Autodesk Inventor part; units mm, degrees
ref_plane "Start Plane" through (0, 0, -4.19) normal (0, 0, 1) x (1, 0, 0)
ref_plane "End Plane" through (0, 0, 265.8983) normal (0, 0, 1) x (1, 0, 0)
ref_plane "Work Plane4" through (10.0091, 3.6912, 287.2885) normal (-0.8617, -0.3178, 0.3957) x (0.468, -0.1962, 0.8617)
ref_plane "Start Plane" through (0, 0, -4.19) normal (0, 0, 1) x (1, 0, 0)
ref_plane "End Plane" through (0, 0, 265.8983) normal (0, 0, 1) x (1, 0, 0)
sketch "Sketch" plane through (0, 0, 0) normal (0, 0, 1) x (1, 0, 0)
  circle A0 centre (0, 0) radius 6.9342
  circle A1 centre (0, 0) radius 10.668
  dimension "d0" = 21.336
  dimension "d1" = 3.7338
extrude "Body" add sketch "Sketch" along normal up to surface (270.0883 mm away) from surface at -4.19
sketch "Sketch3" plane through (0, 0, 0) normal (0, 0, 1) x (1, 0, 0)
  line L0 (0, 0) -> (10, 0)
ref_plane "Work Plane3" through (0, 0, 0) normal (0, -1, 0) x (1, 0, 0)
sketch "Sketch4" plane through (0, 0, 0) normal (0, -1, 0) x (1, 0, 0)
  line L0 (-2, -4.19) -> (12, -4.19)
  line L1 (-2, 265.8983) -> (12, 265.8983)
  dimension "d7" = 270.0883
ref_plane "Work Plane4" through (10.0091, 3.6912, 287.2885) normal (-0.8617, -0.3178, 0.3957) x (0.468, -0.1962, 0.8617)
split "Split1" plane through (10.0091, 3.6912, 287.2885) removes the side toward (-0.8617, -0.3178, 0.3957)
ref_plane "Work Plane5" through (-7.3135, -7.7665, 273.0637) normal (0.4817, 0.5116, 0.7115) x (0.8644, -0.144, -0.4817)
split "Split2" plane through (-7.3135, -7.7665, 273.0637) removes the side toward (0.4817, 0.5116, 0.7115)
ref_plane "Work Plane6" through (7.4386, -7.6468, 269.3352) normal (-0.3751, 0.3856, 0.843) x (0.9237, 0.0785, 0.3751)
split "Split3" plane through (7.4386, -7.6468, 269.3352) removes the side toward (-0.3751, 0.3856, 0.843)
ref_plane "Work Plane7" through (-7.3135, -7.7665, -30.4674) normal (0.647, 0.6871, -0.3305) x (0.3747, -0.664, -0.647)
split "Split4" plane through (-7.3135, -7.7665, -30.4674) removes the side toward (0.647, 0.6871, -0.3305)
ref_plane "Work Plane8" through (-0.1362, -10.6671, -7.916) normal (0.0076, 0.5958, -0.8031) x (0.9997, -0.023, -0.0076)
split "Split5" plane through (-0.1362, -10.6671, -7.916) removes the side toward (0.0076, 0.5958, -0.8031)
ref_plane "Work Plane9" through (10.325, 2.6834, -10.2024) normal (-0.6689, -0.1739, -0.7227) x (-0.6137, -0.4194, 0.6689)
split "Split6" plane through (10.325, 2.6834, -10.2024) removes the side toward (-0.6689, -0.1739, -0.7227)
equation "\"d0\" = G_H"
equation "\"d1\" = G_T"
equation "\"d2\" = G_L"
equation "\"G_H\" = 21.336"
equation "\"G_T\" = 3.7338"
equation "\"G_L\" = 270.08826"
equation "\"G_OFFSET_START\" = 4.18997"
equation "\"G_OFFSET_END\" = 3.36995"
equation "\"d4\" = -G_OFFSET_START"
equation "\"d5\" = G_OFFSET_END + B_L"
equation "\"B_L\" = 262.52833"
properties part number "ANSI - 1/2 x 0.147 - 10.633" material "Steel, Mild"
Work out the finished part from the listing and answer in its coordinate system (mm). Round coordinates to 2 decimals unless told otherwise and drop trailing zeros. Write each loop counter-clockwise with the first axis right and the second up, starting at its lowest first coordinate (ties: lowest second). Pieces come first, ordered by that corner, then holes. Notation, with made-up numbers: (24.25, 40.25) - (49.25, 40.25) arc R6 ccw to (49.25, 45.25) - close; hole circle Ø1 at (70.25, 45.5). An arc over 180 degrees is marked (long way). Return JSON: item names as keys, results as strings. Group by question number.
Q1. Each of these flat-tipped pins is pushed along its axis until it touches: pin 1 Ø3 at (x, z) = (5, 110) entering from -Y; pin 2 Ø10 at (x, y) = (8.5, -2) entering from +Z; pin 3 Ø4 at (y, z) = (-6, 106.5) entering from +X. Where does it stop, or does it pass through?
Q2. The part is cut by section B-B on z = 49. Write down the section's boundary in (x, y).
Q3. The part is cut by section A-A on y = 0. Write down the section's boundary in (x, z), then the cut area to 3 significant figures.
Q4. The mould has two halves that part along Y. Classify faces 1 (the cylindrical face through (3.728, -5.847, 129.125)), 2 (the flat face through (-5.766, -4.613, 246.266)), 3 (the cylindrical face through (10.175, -3.204, 128.963)): released by +Y, released by -Y, zero draft, split by the parting line, or undercut.
Q5. Find the intervals of material crossed by L1, parallel to X at y = 0, z = 65; L2, parallel to Z at x = 4.5, y = -7.25, in increasing order.
Solved:
{
 "1": {"pin 1": "y = -10.08", "pin 2": "z = 263.15", "pin 3": "x = 9.89"},
 "2": {"outline": "circle Ø21.34 at (0, 0); hole circle Ø13.87 at (0, 0)"},
 "3": {"outline": "(-10.67, 9.87) - (-6.93, 6.42) - (-6.93, 247.43) - (-10.67, 239.3) - close; (6.93, 13.57) - (10.67, 20.88) - (10.67, 255.31) - (6.93, 257.83) - close", "area": "1,770 mm²"},
 "4": {"face 1": "undercut", "face 2": "released by -Y", "face 3": "split by the parting line"},
 "5": {"L1": "-10.67 to -6.93, 6.93 to 10.67", "L2": "-2.42 to 264.69"}
}
